Verification items for this drawing (mm, ordinates from the low corner). A direction names the side the tool comes from. Round coordinates to 2 decimals unless told otherwise and drop trailing zeros. Loops run counter-clockwise (first coordinate to the right, second up) from the corner with the lowest first, then second, coordinate; pieces in that order, holes last. Notation, with made-up numbers: (82.25, 5.25) - (101.25, 5.25) arc R10 cw to (101.25, 21.25) - close; hole circle Ø7 at (43.5, 35.25). An arc over 180 degrees is marked (long way). Answer in a Markdown table with one row per item. Add a question column.
(1) Cross-section at A-A on y = 5.5. Enter the section's corners in (x, z).
(2) Access from +Z, -Z, +X, -X, +Y, -Y to the whole of each face (thin tool, end or side, straight path). Record for the marked faces 1, 2 and 3.
(3) Gauge pin test, flat ends, axial feed: pin 1 (0.8 mm diameter, centred on x = 1.5, z = 0.5, fed in from -Y); pin 2 (3 mm diameter, centred on x = 5.5, y = 7, fed in from +Z); pin 3 (10 mm diameter, centred on x = 12.5, y = 10.5, fed in from -Z); pin 4 (8 mm diameter, centred on x = 9.5, z = 6, fed in from +Y). Record the tip position at first contact, or that the pin passes through.
(4) Cross-section at B-B on x = 18. Enter the section's corners in (y, z).
(5) Thickness scan on line 1 along Y through (x, z) = (18.25, 8.5); line 2 along X through (y, z) = (3.25, 2.25); line 3 along Y through (x, z) = (3.5, 13.5). Record the ranges inside material, lowest first.
(6) Cross-section at C-C on z = 2. Enter the section's corners in (x, y), then the cut area to 3 significant figures.
(7) Cross-section at D-D on x = 6. Enter the section's corners in (y, z).
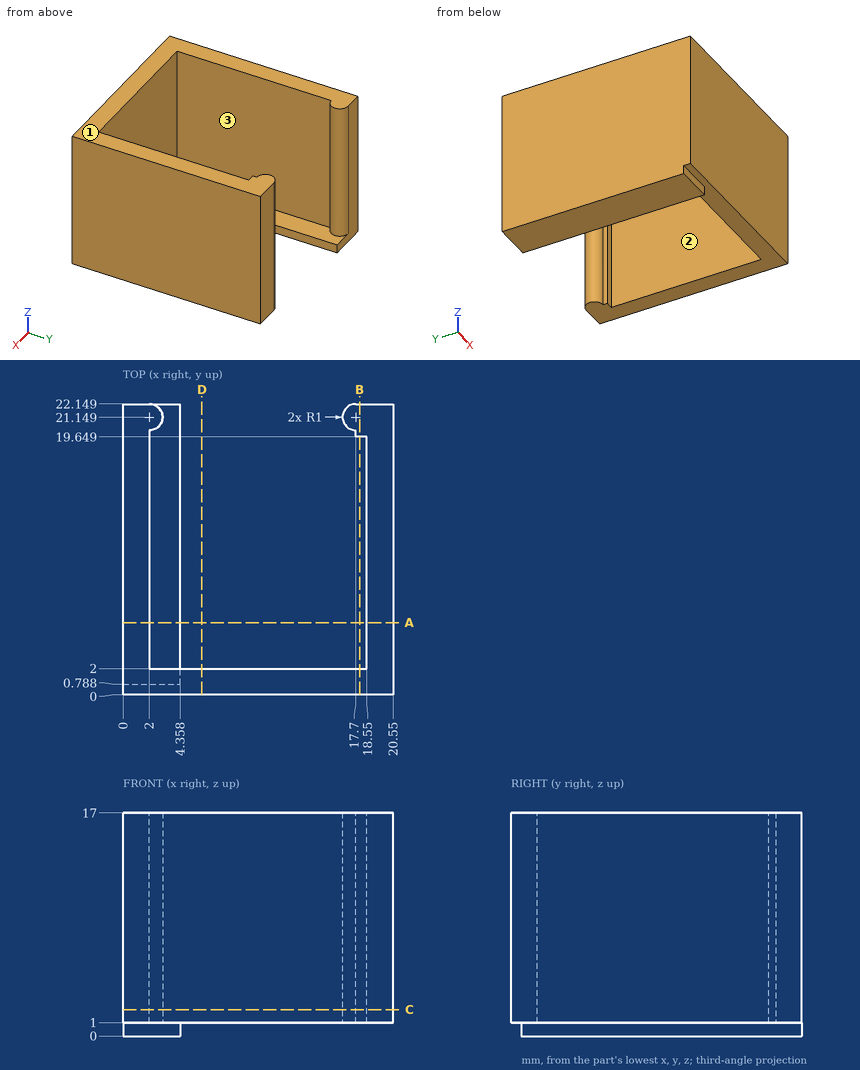
Answers:
| question | item | result |
|---|---|---|
| 1 | outline | (0, 0) - (4.36, 0) - (4.36, 1) - (2, 1) - (2, 17) - (0, 17) - close; (18.55, 1) - (20.55, 1) - (20.55, 17) - (18.55, 17) - close |
| 2 | face 1 | +Z, +X, -X, +Y, -Y |
| 2 | face 2 | +Z, -Z |
| 2 | face 3 | +Z |
| 3 | pin 1 | stops at y = 0.79 |
| 3 | pin 2 | stops at z = 1 |
| 3 | pin 3 | passes through |
| 3 | pin 4 | stops at y = 2 |
| 4 | outline | (0, 1) - (2, 1) - (2, 17) - (0, 17) - close; (19.65, 1) - (22.15, 1) - (22.15, 17) - (19.65, 17) - close |
| 5 | line 1 | y = 0 to 2, 19.65 to 22.15 |
| 5 | line 2 | x = 0 to 2, 18.55 to 20.55 |
| 5 | line 3 | y = 0 to 2 |
| 6 | outline | (0, 0) - (20.55, 0) - (20.55, 22.15) - (17.7, 22.15) arc R1 ccw to (17.7, 20.15) - (17.7, 19.65) - (18.55, 19.65) - (18.55, 2) - (2, 2) - (2, 20.15) arc R1 ccw to (2, 22.15) - (0, 22.15) - close |
| 6 | area | 127 mm^2 |
| 7 | outline | (0, 1) - (2, 1) - (2, 17) - (0, 17) - close |
